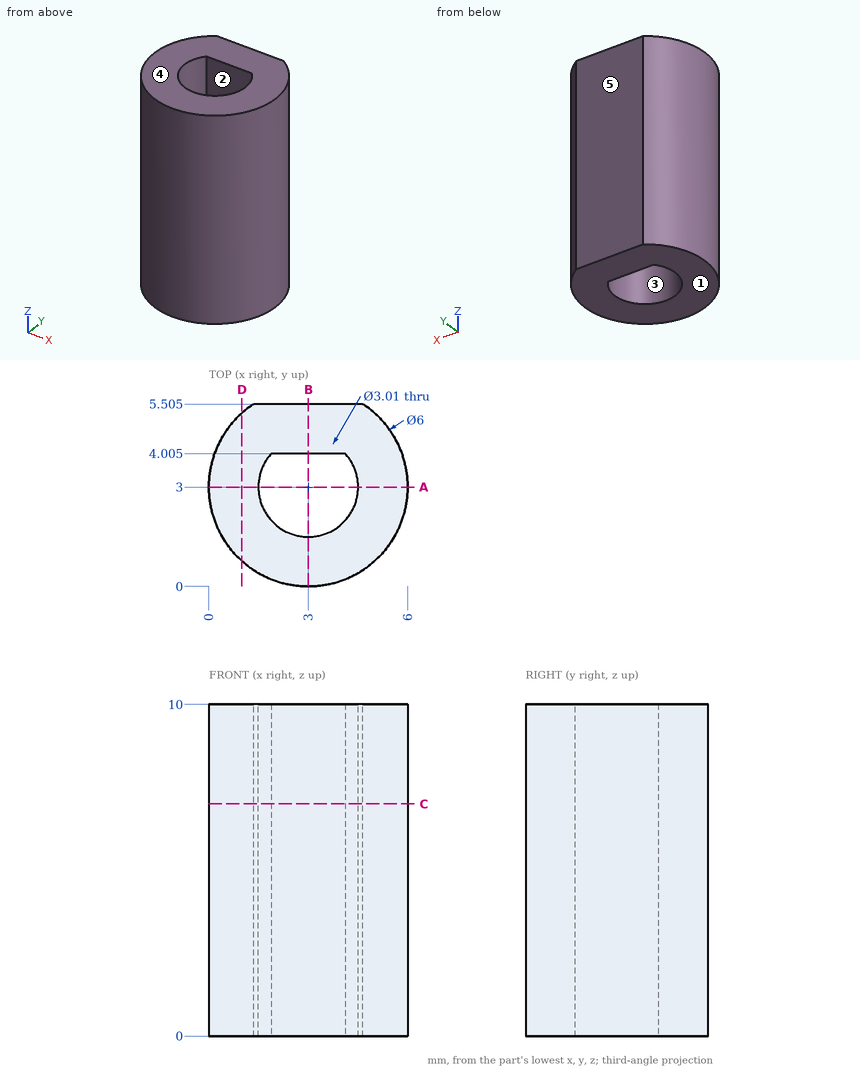
Geometry: see drawing. Coordinates: mm, zero at the bounding-box minimum. A direction names the side the tool comes from. Give positions to 0.01 mm unless a question says otherwise; leave off trailing zeros. Loops run counter-clockwise (first coordinate to the right, second up) from the corner with the lowest first, then second, coordinate; pieces in that order, holes last. Notation, with made-up numbers: (-39, 10.25) - (20, 10.25) arc R15 ccw to (20, 32.25) - close; hole circle Ø7 at (-23.5, 15). An arc over 180 degrees is marked (long way). Use CSV: the item, a comma, the result in double quotes. Start each with the question number.
1. Pin query (flat end, axial travel): pin 1 (2 mm diameter, centred on x = 2.5, z = 3.5, fed in from -Y); pin 2 (1 mm diameter, centred on y = 4.5, z = 5, fed in from +X); pin 3 (1.8 mm diameter, centred on x = 3, y = 3, fed in from +Z). Return the tip coordinate at first contact, or that it passes through.
2. Ray query, L1, parallel to X at y = 3, z = 4.25 (3 decimals); L2, parallel to Y at x = 3, z = 2 (3 decimals); L3, parallel to Y at x = 1.75, z = 7.5 (3 decimals). Return the intervals inside material, ascending.
3. Section B-B (x = 3). Output: boundary loops of the cut face in (y, z) (3 decimals).
4. Section C-C (z = 7). Output: boundary loops of the cut face in (x, y) (3 decimals).
5. Reachability of the marked faces 1 and 2 from +Z, -Z, +X, -X, +Y, -Y: full face, straight path, thin tool, end or side. Return the list, or none.
6. Section D-D (x = 1). Output: boundary loops of the cut face in (y, z), then the cut area to 3 significant figures.
7. Section A-A (y = 3). Output: boundary loops of the cut face in (x, z) (3 decimals).
8. Draft query along Y for the marked faces 3, 4 and 5. Return one class per face: +Y half, -Y half, draft (parallel to the pull), parting line (faces both ways), or undercut.
Response:
1,pin 1,"y = 0"
1,pin 2,"x = 5.83"
1,pin 3,"through"
2,L1,"0 to 1.495, 4.505 to 6"
2,L2,"0 to 1.495, 4.005 to 5.505"
2,L3,"0.273 to 2.162, 3.838 to 5.505"
3,outline,"(0, 0) - (1.495, 0) - (1.495, 10) - (0, 10) - close; (4.005, 0) - (5.505, 0) - (5.505, 10) - (4.005, 10) - close"
4,outline,"(1.349, 5.505) arc R3 ccw (long way) to (4.651, 5.505) - close; hole (1.88, 4.005) arc R1.505 ccw (long way) to (4.12, 4.005) - close"
5,face 1,"-Z, +X, -X, +Y, -Y"
5,face 2,"+Z, -Z"
6,outline,"(0.76, 0) - (5.24, 0) - (5.24, 10) - (0.76, 10) - close"
6,area,"44.7 mm²"
7,outline,"(0, 0) - (1.495, 0) - (1.495, 10) - (0, 10) - close; (4.505, 0) - (6, 0) - (6, 10) - (4.505, 10) - close"
8,face 3,"undercut"
8,face 4,"draft"
8,face 5,"+Y half"
